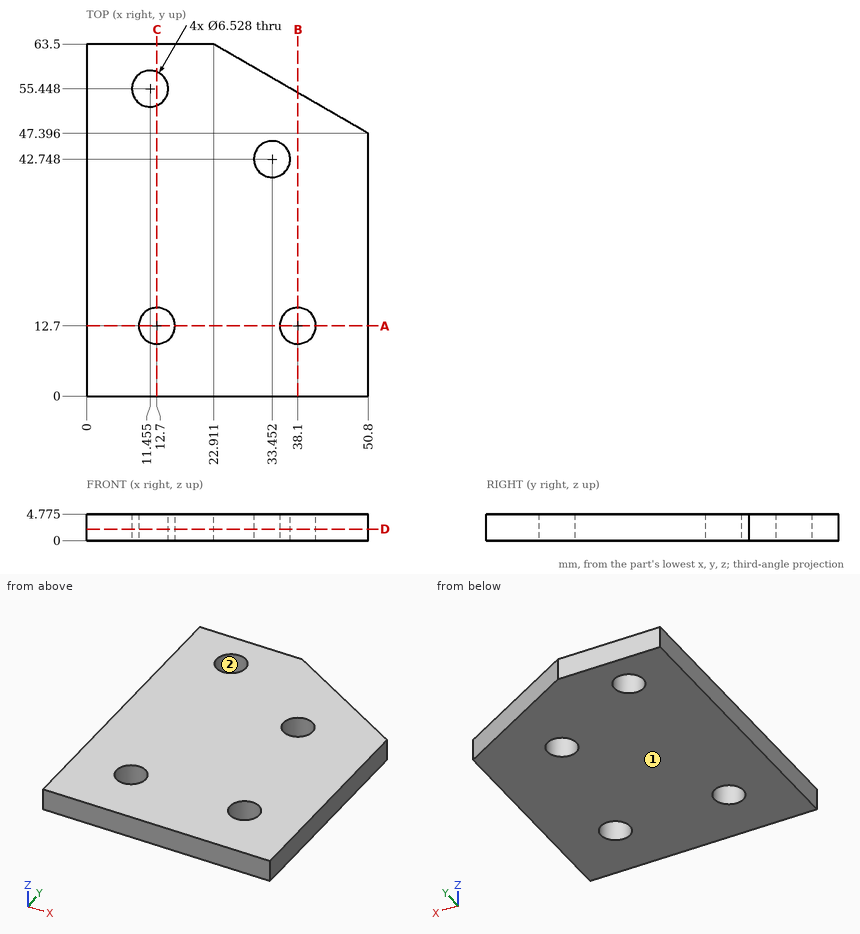
Can you work these out from the drawing? Everything is in mm from the part's minimum corner. Coordinates: 2 decimals unless noted, no trailing zeros. Write each loop counter-clockwise with the first axis right and the second up, starting at its lowest first coordinate (ties: lowest second). Pieces come first, ordered by that corner, then holes. Notation, with made-up numbers: (82, 35.5) -> (109, 35.5) arc R6 ccw to (109, 46.5) -> close; hole circle Ø7 at (21.25, 33.5). An arc over 180 degrees is marked (long way). Write each question's results on one line, items separated by ' | '. Start each with the question number.
Item 1: If we section it at B-B, the plane x = 38.1: Write out the boundary of the cut face in (y, z) (1 decimal).
Item 2: I'm going to push a flat-ended pin straight in: P1, Ø6, axis at x = 33.45, y = 42.75, coming from the +Z side. Where does the tip first touch, or does it pass through?
Item 3: If we section it at C-C, the plane x = 12.7: Write out the boundary of the cut face in (y, z) (1 decimal).
Item 4: Please list where these lines run through material, in increasing order: probe 1 along Y at (x, z) = (12.7, 2.65) (1 decimal); probe 2 along Y at (x, z) = (37, 3) (1 decimal); probe 3 along Y at (x, z) = (10.5, 2.8) (1 decimal).
Item 5: If we section it at A-A, the plane y = 12.7: Write out the boundary of the cut face in (x, z) (1 decimal), and give its area (3 significant figures).
Item 6: Thinking about a two-plate mould opening in X: for the marked faces 1 and 2, which applies, released by +X, released by -X, zero draft, split by the parting line, or undercut?
Item 7: If we section it at D-D, the plane z = 2.1: Write out the boundary of the cut face in (x, y) (1 decimal).
Answer block:
1) outline: (0, 0) -> (9.4, 0) -> (9.4, 4.8) -> (0, 4.8) -> close; (16, 0) -> (54.7, 0) -> (54.7, 4.8) -> (16, 4.8) -> close
2) P1: through
3) outline: (0, 0) -> (9.4, 0) -> (9.4, 4.8) -> (0, 4.8) -> close; (16, 0) -> (52.4, 0) -> (52.4, 4.8) -> (16, 4.8) -> close; (58.5, 0) -> (63.5, 0) -> (63.5, 4.8) -> (58.5, 4.8) -> close
4) probe 1: 0 to 9.4, 16 to 52.4, 58.5 to 63.5 | probe 2: 0 to 9.6, 15.8 to 55.4 | probe 3: 0 to 10.3, 15.1 to 52.3, 58.6 to 63.5
5) outline: (0, 0) -> (9.4, 0) -> (9.4, 4.8) -> (0, 4.8) -> close; (16, 0) -> (34.8, 0) -> (34.8, 4.8) -> (16, 4.8) -> close; (41.4, 0) -> (50.8, 0) -> (50.8, 4.8) -> (41.4, 4.8) -> close | area: 180 mm²
6) face 1: zero draft | face 2: undercut
7) outline: (0, 0) -> (50.8, 0) -> (50.8, 47.4) -> (22.9, 63.5) -> (0, 63.5) -> close; hole circle Ø6.5 at (11.5, 55.4); hole circle Ø6.5 at (12.7, 12.7); hole circle Ø6.5 at (33.5, 42.7); hole circle Ø6.5 at (38.1, 12.7)
